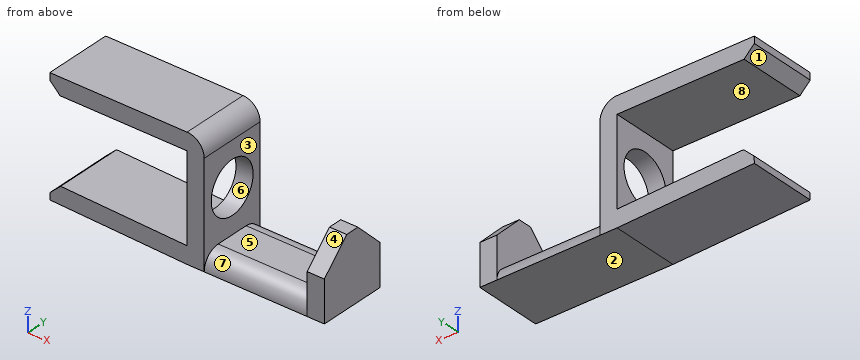
```python
from build123d import *

# Parameters (mm, degrees)
F0_W           = 40
F0_H           = 5
F0_W_2         = 30
F1_DEPTH       = 20
F2_R           = 4.99999
F3_SIZE        = 3
F5_D           = 15
F5_DEPTH       = 20
F5_CBORE_D     = 15
F5_CBORE_DEPTH = 5
F5_TIP         = 4.5064546427
F6_SIZE        = 8


# Not quite as in the source:
# - a fillet or chamfer is up to 0.001 mm smaller than in the source, because OpenCascade refuses the exact size


with BuildPart() as f1:
    # F0 (on Front) → F1 (new body)
    with BuildSketch(Plane.XZ):
        with Locations((-20, 50.4448633795)):
            Rectangle(F0_W, F0_H)
        Polygon((5, 52.9448633795), (0, 52.9448633795), (0, 47.9448633795), (0, 22.6232533795), (0, 17.6205022253), (5, 17.6205022253), (5, 22.6205022253), align=None)
        Polygon((0, 17.6205022253), (0, 22.6232533795), (-39.8342023775, 23.9448633795), (-40, 18.9476130207), align=None)
        with Locations((20, 20.1205022253)):
            Rectangle(F0_W_2, F0_H)
        Polygon((35, 37.6205022253), (35, 22.6205022253), (35, 17.6205022253), (40, 17.6205022253), (40, 37.6205022253), align=None)
    extrude(amount=F1_DEPTH)

    # F2 (radius 5 in the source; OpenCascade refuses exactly that, so slightly less here)
    f2_edges = [f1.edges().sort_by_distance(p)[0] for p in [
        (20, -20, 22.620502),
        (20, 0, 22.620502),
        (5, -10, 52.944863),
    ]]
    fillet(f2_edges, radius=F2_R)

    # F3
    f3_edges = [f1.edges().sort_by_distance(p)[0] for p in [
        (-40, -10, 47.944863),
        (-39.834202, -10, 23.944863),
    ]]
    chamfer(f3_edges, length=F3_SIZE)

    # F5
    with Locations(Plane(origin=(0, 0, 0), x_dir=(0, -1, 0), z_dir=(-1, 0, 0))):
        with Locations((10, 35.2840583795)):
            CounterBoreHole(F5_D / 2, F5_CBORE_D / 2, F5_CBORE_DEPTH, depth=F5_DEPTH)
            with Locations((0, 0, -(F5_DEPTH + F5_TIP / 2))):  # 118° drill point
                Cone(0, F5_D / 2, F5_TIP, mode=Mode.SUBTRACT)

    # F6
    f6_edges = [f1.edges().sort_by_distance(p)[0] for p in [
        (37.5, 0, 37.620502),
        (37.5, -20, 37.620502),
    ]]
    chamfer(f6_edges, length=F6_SIZE)


solid = f1.part
```
The listing builds one solid part. Answer for the finished solid, in the listing's coordinates (mm). Face numbers are marked on the shaded views. A direction names the side the tool comes from. Give positions to 0.01 mm unless a question says otherwise; leave off trailing zeros. Write each loop counter-clockwise with the first axis right and the second up, starting at its lowest first coordinate (ties: lowest second). Pieces come first, ordered by that corner, then holes. Notation, with made-up numbers: M 78,67.5 L 113,67.5 A18 cw 113,71.5 Z; hole C 25,42.25 d7. An arc over 180 degrees is marked long. Write each question's results on one line, items separated by ' | '.
Q1. Consider L1, parallel to X at y = -19, z = 29.5; L2, parallel to X at y = -15, z = 44; L3, parallel to Z at x = 7.5, y = -13.5. Determine where each line is inside the solid, lowest interval first. Write a range as from..to.
Output values:
L1: 0..5, 35..40 | L2: 0..5 | L3: 17.62..22.62
Q2. Section D-D, the plane z = 20 is taken. Write down the section's boundary in (x, y), then the cut area to 3 significant figures.
Output values:
outline: M -39.97,-20 L 5,-20 L 5,-19.4 L 35,-19.4 L 35,-20 L 40,-20 L 40,0 L 35,0 L 35,-0.6 L 5,-0.6 L 5,0 L -39.97,0 Z | area: 1,560 mm2
Q3. For a pull along X with two mould halves and no side action, classify the marked faces 1, 2 and 3 as released by +X, released by -X, zero draft, split by the parting line, or undercut.
Output values:
face 1: released by -X | face 2: zero draft | face 3: undercut
Q4. Flat-ended cylindrical pins translate along their axes: P1, Ø6, axis at y = -8, z = 35.5, coming from the -X side; P2, Ø3, axis at y = -9.5, z = 46.5, coming from the +X side; P3, Ø8, axis at x = 15, y = -8, coming from the +Z side; P4, Ø8, axis at x = -12, z = 43, coming from the -Y side. Find the tip coordinate at first contact, or state that the pin passes through.
Output values:
P1: x = 35 | P2: x = 5 | P3: z = 22.62 | P4: through
Q5. Section A-A, the plane y = -10 is taken. Write down the section's boundary in (x, z), then the cut area to 3 significant figures.
Output values:
outline: M -40,18.95 L 0,17.62 L 40,17.62 L 40,37.62 L 35,37.62 L 35,22.62 L 5,22.62 L 5,27.78 L 0,27.78 L 0,22.62 L -36.84,23.85 L -39.93,20.95 Z; M -40,50.94 L -37,47.94 L 0,47.94 L 0,42.78 L 5,42.78 L 5,47.94 A5 ccw 0,52.94 L -40,52.94 Z | area: 737 mm2
Q6. Section C-C, the plane y = -1.5 is taken. Write down the section's boundary in (x, z), then the cut area to 3 significant figures.
Output values:
outline: M -40,18.95 L 0,17.62 L 40,17.62 L 40,31.12 L 35,31.12 L 35,21.19 L 5,21.19 L 5,47.94 A5 ccw 0,52.94 L -40,52.94 L -40,50.94 L -37,47.94 L 0,47.94 L 0,22.62 L -36.84,23.85 L -39.93,20.95 Z | area: 737 mm2
Q7. A tool of negligible diameter and unlimited length cuts with its end or side. For the marked faces 4, 5, 6, 7 and 8, from which of +Z, -Z, +X, -X, +Y, -Y can it reach the whole face along a straight path? Write none if from no direction.
Output values:
face 4: +Z, +X, -Y | face 5: +Z, +Y, -Y | face 6: -X | face 7: +Z, -Y | face 8: -X, +Y, -Y
Q8. Section B-B, the plane x = -23.5 is taken. Write down the section's boundary in (y, z), then the cut area to 3 significant figures.
Output values:
outline: M -20,18.4 L 0,18.4 L 0,23.4 L -20,23.4 Z; M -20,47.94 L 0,47.94 L 0,52.94 L -20,52.94 Z | area: 200 mm2
